Check sheet for the modelled part. Datum: model origin and axes. Units: mm. Face numbers are marked on the shaded views. A direction names the side the tool comes from. Coordinates: 2 decimals unless noted, no trailing zeros. Order: outer loops, then holes, each group sorted by start corner. A loop starts at its lowest first (then second) coordinate and runs counter-clockwise, first axis right, second up. Notation, with made-up numbers: (2, -14) -> (27, -14) arc R20 cw to (27, 23) -> close; hole circle Ø10 at (29.25, 38.25). An arc over 180 degrees is marked (long way). Put each result on its own line as item: value. Start each with the question number.
```python
from build123d import *

# Parameters (mm, degrees)
SKETCH1_W           = 70
SKETCH1_H           = 12
BOSS_EXTRUDE1_DEPTH = 10
BOSS_EXTRUDE2_DEPTH = 12
SKETCH3_R           = 2
CUT_EXTRUDE1_DEPTH  = 12


with BuildPart() as part:
    # Sketch1 → Boss-Extrude1 (new body)
    with BuildSketch(Plane(origin=(0, 0, 0), x_dir=(0, 0, -1), z_dir=(1, 0, 0))):
        Rectangle(SKETCH1_W, SKETCH1_H)
    extrude(amount=BOSS_EXTRUDE1_DEPTH)

    # Sketch2 → Boss-Extrude2 (add)
    with BuildSketch(Plane(origin=(0, 6, 0), x_dir=(1, 0, 0), z_dir=(0, 1, 0))):
        with BuildLine():
            add(Edge.make_bspline(
                [(10, -15), (30.647953976, -28.668903478), (50.105658194, -9.868255971)],
                knots=[0, 0, 0, 1, 1, 1], degree=2))
            Line((10, -15), (10, -20.717636889))
            add(Edge.make_bspline(
                [(10, -20.717636889), (21.360270844, -26.451655212), (47.984708218, -26.799299217), (50.105658194, -9.868255971)],
                knots=[0, 0, 0, 0, 1, 1, 1, 1], degree=3))
        make_face()
        with BuildLine():
            Line((10, 20.717636889), (10, 15))
            add(Edge.make_bspline(
                [(10, 15), (30.647953976, 28.668903478), (50.105658194, 9.868255971)],
                knots=[0, 0, 0, 1, 1, 1], degree=2))
            add(Edge.make_bspline(
                [(10, 20.717636889), (21.360270844, 26.451655212), (47.984708218, 26.799299217), (50.105658194, 9.868255971)],
                knots=[0, 0, 0, 0, 1, 1, 1, 1], degree=3))
        make_face()
    extrude(amount=-BOSS_EXTRUDE2_DEPTH)

    # Sketch3 → Cut-Extrude1 (cut)
    with BuildSketch(Plane.ZY):
        Circle(SKETCH3_R)
    extrude(amount=-CUT_EXTRUDE1_DEPTH, mode=Mode.SUBTRACT)


solid = part.part
```
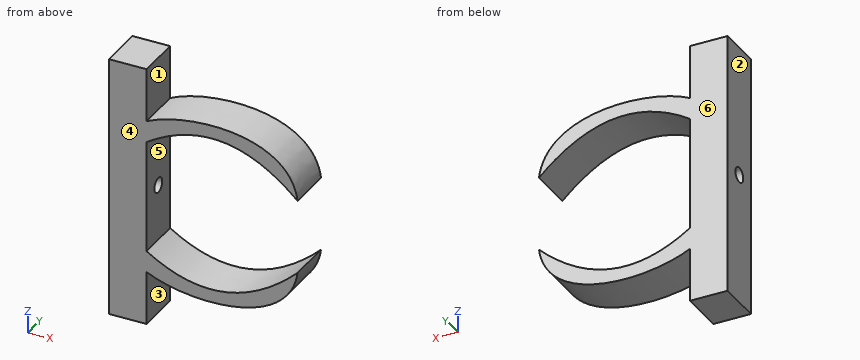
1) Scan lines: line 1 along Y through (x, z) = (8.25, 0); line 2 along Z through (x, y) = (25.5, 0); line 3 along Z through (x, y) = (22, -4.75). Record each from-to range of solid material in increasing order. Write a range as [from, to].
2) Access from +Z, -Z, +X, -X, +Y, -Y to the whole of each face (thin tool, end or side, straight path). Record for the marked faces 5 and 6.
3) Gauge pin test, flat ends, axial feed: pin 1 (1 mm diameter, centred on x = 22, y = -1.5, fed in from -Z); pin 2 (6 mm diameter, centred on y = 3, z = -4.5, fed in from +X); pin 3 (4 mm diameter, centred on x = 25, y = -4.5, fed in from +Z). Record the tip position at first contact, or that the pin passes through.
4) Sectioned sample at A-A (z = 0). Record the boundary of the cut face in (x, y).
5) Sectioned sample at B-B (z = -25). Record the boundary of the cut face in (x, y).
6) Mould release check, pull along X, two halves, no side actions. Record for the marked faces 1, 2, 3 and 4: +X half, -X half, draft (parallel to the pull), parting line (faces both ways), or undercut.
Entries:
1. line 1: y = [-6, -2], [2, 6]
1. line 2: z = [-24.24, -20.7], [20.7, 24.24]
1. line 3: z = [-23.98, -20.22], [20.22, 23.98]
2. face 5: +Y, -Y
2. face 6: +Z, -Z, +X, -X, +Y
3. pin 1: stops at z = -24.03
3. pin 2: stops at x = 10
3. pin 3: stops at z = 24.27
4. outline: (0, -6) -> (10, -6) -> (10, -2) -> (0, -2) -> close; (0, 2) -> (10, 2) -> (10, 6) -> (0, 6) -> close
5. outline: (0, -6) -> (10, -6) -> (10, 6) -> (0, 6) -> close
6. face 1: undercut
6. face 2: -X half
6. face 3: undercut
6. face 4: draft
